Here's how the part is built. I have some questions about the finished solid (model axes, mm). A direction names the side the tool comes from. Coordinates: 2 decimals unless noted, no trailing zeros. Use a Markdown table: item, result. Add a question column.
Item 1: Will these pins go through, and if not, where does the flat tip stop? pin 1 Ø1.4 at (y, z) = (2, -1) entering from -X; pin 2 Ø0.8 at (x, y) = (4.5, 1.5) entering from +Z (3 decimals); pin 3 Ø1.4 at (y, z) = (1.5, -1) entering from +X.
Item 2: Imagine slicing it at A-A, the plane y = 1.45. Count the separate pieces of the cut face and the enclosed holes in it, and give its area (3 significant figures).
Item 3: If I drill on line 1 along X through (y, z) = (0.3, -3.25); line 2 along Z through (x, y) = (33.5, 1.9); line 3 along X through (y, z) = (0.65, -1.25) (3 decimals), over which ranges is the centre line in solid material (lowest first)? Write a range as from..to.
Item 4: If we mould it in two halves opening along X, with no side actions, what happens to faces 1 (the flat face through (29, 2.794, -3)), 2 (the cylindrical face through (57.618, 1.417, -5.626)), 3 (the flat face through (3.175, 1, -2))? For each: pulls with the +X half, pulls with the -X half, needs draft (parallel to the pull), parting line crosses it, or undercut.
Item 5: On a 3-axis mill with a long thin cutter (end or side, diameter ignored), from which of +Z, -Z, +X, -X, +Y, -Y can I reach the whole of each face in a straight line? I mean faces 4 (the flat face through (41, 1, 0)), 5 (the flat face through (23.838, 1, -2)). Say none if no direction works.
```python
from build123d import *

# Parameters (mm, degrees)
BOSS_EXTRUDE1_DEPTH = 2.794
SKETCH2_R           = 0.9525
CUT_EXTRUDE1_DEPTH  = 59.792605897
FILLET2_R           = 2.54


with BuildPart() as part:
    # Sketch1 → Boss-Extrude1 (new body)
    with BuildSketch(Plane(origin=(0, 0, 0), x_dir=(1, 0, 0), z_dir=(0, 1, 0))):
        Polygon((0, 0), (3.175, 0), (3.175, 3.175), (5.969, 3.175), (5.969, 0), (23.837859958, 0), (23.837859958, 3.175), (26.631859958, 3.175), (26.631859958, 0), (58.381859958, 0), (58.381859958, 6.35), (0, 6.35), align=None)
    extrude(amount=BOSS_EXTRUDE1_DEPTH)

    # Sketch2 → Cut-Extrude1 (cut, through all)
    with BuildSketch(Plane(origin=(0, 2.794, 0), x_dir=(1, 0, 0), z_dir=(0, 1, 0))):
        with Locations(Location((55.206859958, 3.175, 0), (0, 0, 270))):
            Circle(SKETCH2_R)
        with Locations(Location((34.206859958, 3.175, 0), (0, 0, 270))):
            Circle(SKETCH2_R)
    extrude(amount=-CUT_EXTRUDE1_DEPTH, mode=Mode.SUBTRACT)

    # Fillet2
    fillet2_edges = [part.edges().sort_by_distance(p)[0] for p in [
        (58.381859958, 1.397, -6.35),
        (58.381859958, 1.397, 0),
    ]]
    fillet(fillet2_edges, radius=FILLET2_R)


solid = part.part
```
Ans:
| question | item | result |
|---|---|---|
| 1 | pin 1 | stops at x = 0 |
| 1 | pin 2 | stops at z = -3.175 |
| 1 | pin 3 | stops at x = 58.24 |
| 2 | separate pieces | 1 |
| 2 | enclosed holes | 2 |
| 2 | area | 345 mm^2 |
| 3 | line 1 | x = 0..33.26, 35.16..54.26, 56.16..58.38 |
| 3 | line 2 | z = -6.35..-3.81, -2.54..0 |
| 3 | line 3 | x = 0..3.175, 5.969..23.838, 26.632..58.03 |
| 4 | face 1 | needs draft |
| 4 | face 2 | pulls with the +X half |
| 4 | face 3 | undercut |
| 5 | face 4 | +Z, +X, -X, +Y, -Y |
| 5 | face 5 | +Z, +Y, -Y |
